Autodesk Inventor part; units mm, degrees
ref_plane "YZ Plane" through (0, 0, 0) normal (1, 0, 0) x (0, 1, 0)
ref_plane "XZ Plane" through (0, 0, 0) normal (0, 1, 0) x (-1, 0, 0)
sketch "Skizze1" plane through (0, 0, 0) normal (0, 0, 1) x (1, 0, 0)
  circle A0 centre (0, 0) radius 30
  circle A1 centre (0, 0) radius 27
  dimension "d0" = 60
  dimension "d1" = 54
extrude "Extrusion1" add sketch "Skizze1" along normal mid plane 25
ref_plane "Arbeitsebene1" through (0, 0, 6) normal (0, 0, 1) x (1, 0, 0)
sketch "Skizze2" plane through (0, 0, 6) normal (0, 0, 1) x (1, 0, 0)
  line L0 (0, 39.0372) -> (0, -37.5893) construction
  circle A0 centre (0, 0) radius 30 construction
  point P0 (0, 30)
ref_plane "Arbeitsebene2" through (0, 30, 6) normal (0, 1, 0) x (-1, 0, 0)
sketch "Skizze3" plane through (0, 30, 6) normal (0, 1, 0) x (-1, 0, 0)
  circle A0 centre (0, 0) radius 1.75
  point P0 (0, -6)
  dimension "d5" = 3.5
extrude "Extrusion2" cut sketch "Skizze3" against normal blind 5
pattern_circular "Runde Anordnung1" count 3 over 360 about axis through (0, 0, -10) along (0, 0, 1) of "Extrusion2"
mirror "Spiegeln1" about plane through (0, 0, 0) normal (0, 0, 1) of "Extrusion2", "Runde Anordnung1"
chamfer "Fase1" distance 0.5 angle 45 2 edges at (-27, 0, 12.5) (-27, 0, -12.5)
sketch "Skizze5" plane through (0, 0, 0) normal (0, 0, 1) x (1, 0, 0)
  circle A0 centre (0, 0) radius 27
  line L0 (-4.3192, -1.9196) -> (5.9435, -1.9196)
  line L1 (5.9435, -1.9196) -> (5.9435, 1.6981)
  line L2 (5.9435, 1.6981) -> (-4.3192, 1.6981)
  line L3 (-4.3192, 1.6981) -> (-4.3192, -1.9196)
extrude "Extrusion4" add sketch "Skizze5" along normal mid plane 4
sketch "Skizze4" plane through (0, 0, 0) normal (0, 0, 1) x (1, 0, 0)
  line L0 (0, 34.5644) -> (0, -38.5024) construction
  line L1 (-38.0901, 0) -> (52.3904, 0) construction
  line L2 (-34.7368, 16.5) -> (36.624, 16.5) construction
  line L3 (-36.0898, -16.5) -> (37.8594, -16.5) construction
  line L4 (16.5, 35.2115) -> (16.5, -32.6782) construction
  line L5 (-16.5, 34.5644) -> (-16.5, -34.6196) construction
  circle A0 centre (-16.5, 16.5) radius 1.75
  circle A1 centre (16.5, 16.5) radius 1.75
  circle A2 centre (-16.5, -16.5) radius 1.75
  circle A3 centre (16.5, -16.5) radius 1.75
  circle A4 centre (-16.5, 16.5) radius 3.6693
  circle A5 centre (16.5, 16.5) radius 3.7169
  circle A6 centre (16.5, -16.5) radius 3.6667
  circle A7 centre (-16.5, -16.5) radius 3.6675
  point P0 (0, 0)
  dimension "d14" = 33
  dimension "d15" = 33
  dimension "d16" = 3.5
  dimension "d17" = 3.5
  dimension "d18" = 3.5
  dimension "d19" = 3.5
extrude "Extrusion3" add sketch "Skizze4" along normal mid plane 4
extrude "Extrusion5" cut sketch "Skizze4" against normal mid plane 4 contours A0 | A1 | A2 | A3
sketch "Skizze6" plane through (0, 0, 0) normal (0, 0, 1) x (1, 0, 0)
  circle A0 centre (0, 0) radius 31
  circle A1 centre (0, 0) radius 29
  dimension "d27" = 62
  dimension "d28" = 58
extrude "Extrusion6" add sketch "Skizze6" along normal mid plane 1
ref_plane "Arbeitsebene3" through (0, 0, -6) normal (0, 0, 1) x (1, 0, 0)
ref_plane "Arbeitsebene4" through (0, 30, -6) normal (0, -1, 0) x (-1, 0, 0)
properties part number "_3D-Druck"
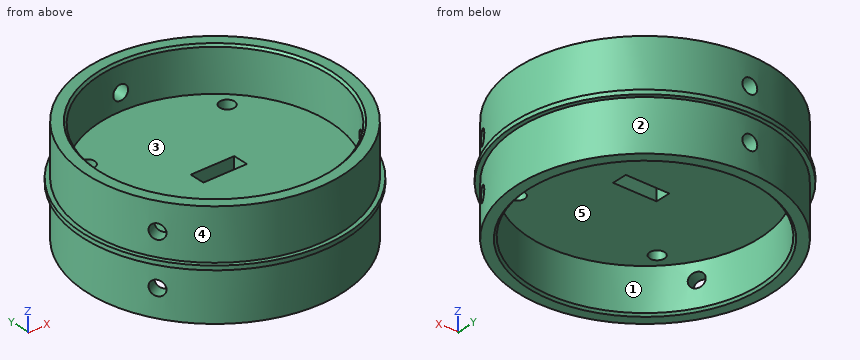
Can you work these out from the model? Positions are in its coordinate system, mm. Face numbers are marked on the shaded views. A direction names the side the tool comes from. Round coordinates to 2 decimals unless told otherwise and drop trailing zeros. Order: outer loops, then holes, each group sorted by start corner. A loop starts at its lowest first (then second) coordinate and runs counter-clockwise, first axis right, second up.
(1) If I drill on L1, parallel to Z at x = 0, y = 28.9; L2, parallel to Y at x = -16.5, z = -0.9; L3, parallel to Z at x = -23, y = -8.5, over which ranges is the centre line in solid material (lowest first)?
Results are:
L1: z = -12.5 to -7.75, -4.25 to 4.25, 7.75 to 12.5
L2: y = -25.05 to -18.25, -14.75 to 14.75, 18.25 to 25.05
L3: z = -2 to 2
(2) We'd pull the mould along Y, two halves only. Please class the marked faces 1, 2 and 3: +Y half, -Y half, draft (parallel to the pull), parting line (faces both ways), or undercut.
Results are:
face 1: undercut
face 2: parting line
face 3: undercut
(3) If we section it at C-C (x = 0): Count the separate pieces of the cut face and the enclosed holes in it, plus the area to 3 significant figures.
Results are:
separate pieces: 4
enclosed holes: 0
area: 332 mm2
(4) On a 3-axis mill with a long thin cutter (end or side, diameter ignored), from which of +Z, -Z, +X, -X, +Y, -Y can I reach the whole of each face in a straight line? I mean the marked faces 4 and 5. Say none if no direction works.
Results are:
face 4: +Z
face 5: -Z
(5) If we section it at A-A (z = -6): Please give me the cut outline in (x, y).
Results are:
outline: (-26.81, -13.46) - (-24.21, -11.96) arc R27 cw to (-1.75, 26.94) - (-1.75, 29.95) arc R30 ccw to start; (-25.06, -16.49) arc R30 ccw to (25.06, -16.49) - (22.46, -14.99) arc R27 cw to (-22.46, -14.99) - close; (1.75, 26.94) arc R27 cw to (24.21, -11.96) - (26.81, -13.46) arc R30 ccw to (1.75, 29.95) - close
(6) If we section it at B-B (z = 9.75): Please give me the cut outline in (x, y).
Results are:
outline: circle Ø60 at (0, 0); hole circle Ø54 at (0, 0)
(7) I'm going to push flat-ended pins straight in: pin 1 (2 mm diameter, centred on x = -8, y = 5.5, fed in from +Z); pin 2 (3 mm diameter, centred on x = 2, z = 0.5, fed in from -Y); pin 3 (18.5 mm diameter, centred on x = -9.5, y = -5, fed in from -Z). Where does each tip first touch, or does it pass through?
Results are:
pin 1: stops at z = 2
pin 2: stops at y = -31
pin 3: stops at z = -2
